```python
from build123d import *

# Parameters (mm, degrees)
SKETCH1_R           = 15
BOSS_EXTRUDE1_DEPTH = 3
BOSS_EXTRUDE2_DEPTH = 40
CHAMFER1_SIZE       = 3
SKETCH4_R           = 10
BOSS_EXTRUDE3_DEPTH = 35
SKETCH6_W           = 20
SKETCH6_H           = 10
CUT_EXTRUDE1_DEPTH  = 5
SKETCH8_R           = 1.5
CUT_EXTRUDE3_DEPTH  = 4


with BuildPart() as part:
    # Sketch1 → Boss-Extrude1 (new body)
    with BuildSketch(Plane.XY):
        with BuildLine():
            Line((-123, 116), (-123, -25))
            ThreePointArc((-123, -25), (-118.606601718, -35.606601718), (-108, -40))
            Line((-108, -40), (160, -40))
            ThreePointArc((160, -40), (170.606601718, -35.606601718), (175, -25))
            Line((175, -25), (175, 116))
            ThreePointArc((175, 116), (170.606601718, 126.606601718), (160, 131))
            Line((160, 131), (-108, 131))
            ThreePointArc((-108, 131), (-118.606601718, 126.606601718), (-123, 116))
        make_face()
        Circle(SKETCH1_R, mode=Mode.SUBTRACT)
        with Locations((-47, 75)):
            Circle(SKETCH1_R, mode=Mode.SUBTRACT)
        with Locations((-15, 56)):
            Circle(SKETCH1_R, mode=Mode.SUBTRACT)
        with Locations((-83, 75)):
            Circle(SKETCH1_R, mode=Mode.SUBTRACT)
        with Locations((31, 76)):
            Circle(SKETCH1_R, mode=Mode.SUBTRACT)
        with Locations((65, 91)):
            Circle(SKETCH1_R, mode=Mode.SUBTRACT)
        with Locations((101, 91)):
            Circle(SKETCH1_R, mode=Mode.SUBTRACT)
        with Locations((24, 36)):
            Circle(SKETCH1_R, mode=Mode.SUBTRACT)
        with Locations((58, 51)):
            Circle(SKETCH1_R, mode=Mode.SUBTRACT)
        with Locations((94, 51)):
            Circle(SKETCH1_R, mode=Mode.SUBTRACT)
        with Locations((135, 81)):
            Circle(SKETCH1_R, mode=Mode.SUBTRACT)
        with Locations((128, 41)):
            Circle(SKETCH1_R, mode=Mode.SUBTRACT)
    extrude(amount=-BOSS_EXTRUDE1_DEPTH)

    # Sketch2 → Boss-Extrude2 (add)
    with BuildSketch(Plane(origin=(0, 0, -3), x_dir=(-1, 0, 0), z_dir=(0, 0, -1))):
        with BuildLine():
            Line((123, -25), (123, 116))
            ThreePointArc((123, 116), (118.606601718, 126.606601718), (108, 131))
            Line((108, 131), (-160, 131))
            ThreePointArc((-160, 131), (-170.606601718, 126.606601718), (-175, 116))
            Line((-175, 116), (-175, -25))
            ThreePointArc((-175, -25), (-170.606601718, -35.606601718), (-160, -40))
            Line((-160, -40), (108, -40))
            ThreePointArc((108, -40), (118.606601718, -35.606601718), (123, -25))
        make_face()
        with BuildLine():
            Line((118, -25), (118, 116))
            ThreePointArc((118, 116), (115.071067812, 123.071067812), (108, 126))
            Line((108, 126), (-160, 126))
            ThreePointArc((-160, 126), (-167.071067812, 123.071067812), (-170, 116))
            Line((-170, 116), (-170, -25))
            ThreePointArc((-170, -25), (-167.071067812, -32.071067812), (-160, -35))
            Line((-160, -35), (108, -35))
            ThreePointArc((108, -35), (115.071067812, -32.071067812), (118, -25))
        make_face(mode=Mode.SUBTRACT)
    extrude(amount=BOSS_EXTRUDE2_DEPTH)

    # Chamfer1
    chamfer1_edges = [part.edges().sort_by_distance(p)[0] for p in [
        (26, 131, 0),
        (170.606601718, 126.606601718, 0),
        (175, 45.5, 0),
        (170.606601718, -35.606601718, 0),
        (26, -40, 0),
        (-118.606601718, -35.606601718, 0),
        (-123, 45.5, 0),
        (-118.606601718, 126.606601718, 0),
    ]]
    chamfer(chamfer1_edges, length=CHAMFER1_SIZE)

    # Sketch4 → Boss-Extrude3 (add)
    with BuildSketch(Plane(origin=(0, 0, -3), x_dir=(-1, 0, 0), z_dir=(0, 0, -1))):
        with Locations((-160, 116)):
            Circle(SKETCH4_R)
        with Locations((108, 116)):
            Circle(SKETCH4_R)
        with Locations((-160, -25)):
            Circle(SKETCH4_R)
        with Locations((108, -25)):
            Circle(SKETCH4_R)
    extrude(amount=BOSS_EXTRUDE3_DEPTH)

    # Sketch6 → Cut-Extrude1 (cut)
    with BuildSketch(Plane(origin=(0, 131, 0), x_dir=(1, 0, 0), z_dir=(0, 1, 0))):
        with Locations((-68, 28)):
            Rectangle(SKETCH6_W, SKETCH6_H)
    extrude(amount=-CUT_EXTRUDE1_DEPTH, mode=Mode.SUBTRACT)

    # Sketch8 → Cut-Extrude3 (cut)
    with BuildSketch(Plane(origin=(0, 0, -38), x_dir=(-1, 0, 0), z_dir=(0, 0, -1))):
        with Locations((-160, 116)):
            Circle(SKETCH8_R)
        with Locations((108, 116)):
            Circle(SKETCH8_R)
        with Locations((-160, -25)):
            Circle(SKETCH8_R)
        with Locations((108, -25)):
            Circle(SKETCH8_R)
    extrude(amount=-CUT_EXTRUDE3_DEPTH, mode=Mode.SUBTRACT)


solid = part.part
```
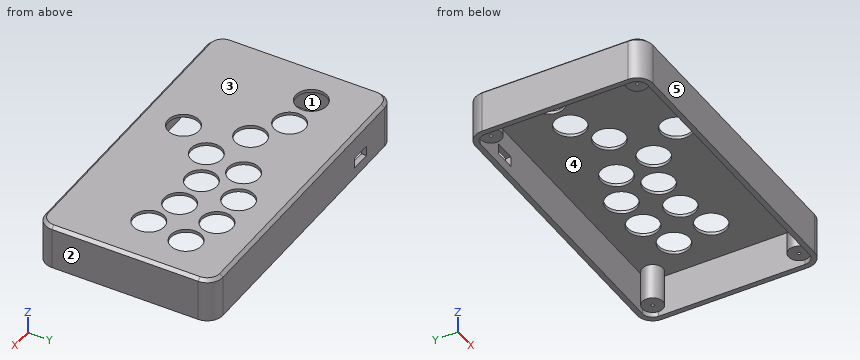
Read the model definition and answer for the solid it produces. Units are mm, in the model's axes. Face numbers are marked on the shaded views. A direction names the side the tool comes from. Coordinates: 2 decimals unless noted, no trailing zeros. Loops run counter-clockwise (first coordinate to the right, second up) from the corner with the lowest first, then second, coordinate; pieces in that order, holes last. Notation, with made-up numbers: (42, -4.5) - (75, -4.5) arc R17 cw to (75, 22.5) - close; hole circle Ø11 at (69, 46.5). An arc over 180 degrees is marked (long way). Answer in a Markdown table with one row per item.
1. Find section D-D, the plane y = 84.5. Count the separate pieces of the cut face and the enclosed holes in it, then the cut area to 3 significant figures.
Conclusion:
| item | result |
|---|---|
| separate pieces | 7 |
| enclosed holes | 0 |
| area | 822 mm² |
2. Straight lines are drawn through the part: line 1 (X direction, y = 4.5, z = -7.5); line 2 (Y direction, x = 146.5, z = -24.5); line 3 (Z direction, x = 110, y = -11.5). For each, find the intervals that lie inside material, in ascending order.
Conclusion:
| item | result |
|---|---|
| line 1 | x = -123 to -118, 170 to 175 |
| line 2 | y = -40 to -35, 126 to 131 |
| line 3 | z = -3 to 0 |
3. Which of the six approach directions +Z, -Z, +X, -X, +Y, -Y give full straight-line access (tool end or side, diameter ignored) to the marked faces 4 and 5?
Conclusion:
| item | result |
|---|---|
| face 4 | -Z |
| face 5 | +Z, -Z, +X, -X, -Y |
4. Find section C-C, the plane z = -8.5. Write down the section's boundary in (x, y).
Conclusion:
| item | result |
|---|---|
| outline | (-123, -25) arc R15 ccw to (-108, -40) - (160, -40) arc R15 ccw to (175, -25) - (175, 116) arc R15 ccw to (160, 131) - (-108, 131) arc R15 ccw to (-123, 116) - close; hole (-118, -25) arc R10 cw (long way) to (-108, -35) - (160, -35) arc R10 cw (long way) to (170, -25) - (170, 116) arc R10 cw (long way) to (160, 126) - (-108, 126) arc R10 cw (long way) to (-118, 116) - close |
5. Given pin 1 (5 mm diameter, centred on x = 20, y = 50.5, fed in from -Z); pin 2 (3.5 mm diameter, centred on x = 160, y = 116.5, fed in from -Z), each flat-ended and moving along its own axis, determine where each tip first touches the part or whether it passes through.
Conclusion:
| item | result |
|---|---|
| pin 1 | stops at z = -3 |
| pin 2 | stops at z = -38 |
6. Determine the mould class of the marked faces 1, 2 and 3 for opening direction X: +X half, -X half, draft (parallel to the pull), parting line (faces both ways), or undercut.
Conclusion:
| item | result |
|---|---|
| face 1 | undercut |
| face 2 | +X half |
| face 3 | draft |
7. Find section A-A, the plane y = 0. Write down the section's boundary in (x, z), then the cut area to 4 significant figures.
Conclusion:
| item | result |
|---|---|
| outline | (-123, -43) - (-118, -43) - (-118, -3) - (-15, -3) - (-15, 0) - (-120, 0) - (-123, -3) - close; (15, -3) - (170, -3) - (170, -43) - (175, -43) - (175, -3) - (172, 0) - (15, 0) - close |
| area | 1,195 mm² |
8. Find section B-B, the plane x = -47. Write down the section's boundary in (y, z).
Conclusion:
| item | result |
|---|---|
| outline | (-40, -43) - (-35, -43) - (-35, -3) - (60, -3) - (60, 0) - (-37, 0) - (-40, -3) - close; (90, -3) - (126, -3) - (126, -43) - (131, -43) - (131, -3) - (128, 0) - (90, 0) - close |
